Work out the finished part from the listing and answer in its coordinate system (mm). Face numbers are marked on the shaded views. Coordinates: 2 decimals unless noted, no trailing zeros. Loops run counter-clockwise (first coordinate to the right, second up) from the corner with the lowest first, then second, coordinate; pieces in that order, holes last.
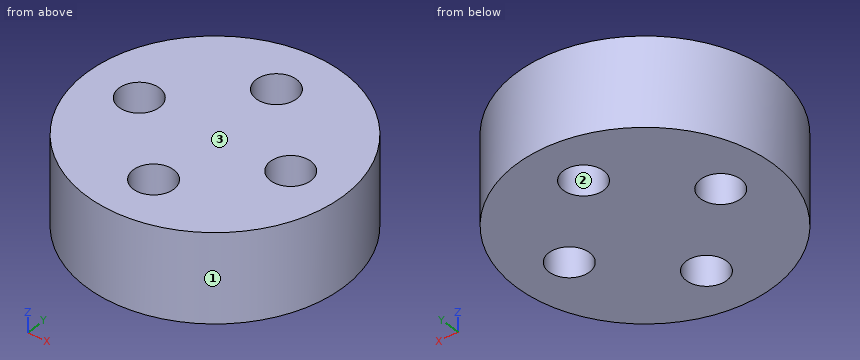
Autodesk Inventor part; units mm, degrees
ref_plane "YZ Plane" through (0, 0, 0) normal (1, 0, 0) x (0, 1, 0)
ref_plane "XZ Plane" through (0, 0, 0) normal (0, 1, 0) x (-1, 0, 0)
ref_plane "XY Plane" through (0, 0, 0) normal (0, 0, 1) x (1, 0, 0)
sketch "스케치1" plane through (0, 0, 0) normal (0, 0, 1) x (1, 0, 0)
  circle A0 centre (0, 0) radius 10.15
  line L0 (0, 0) -> (-6, 0)
  circle A1 centre (-6, 0) radius 1.6
  line L1 (0, 0) -> (0, 6)
  circle A2 centre (0, 6) radius 1.6
  line L2 (0, 0) -> (0, -6)
  circle A3 centre (0, -6) radius 1.6
  line L3 (0, 0) -> (6, 0)
  circle A4 centre (6, 0) radius 1.6
  dimension "d2" = 6
  dimension "d3" = 3.2
  dimension "d7" = 6
  dimension "d8" = 3.2
  dimension "d9" = 6
  dimension "d10" = 3.2
  dimension "d11" = 6
  dimension "d12" = 3.2
  dimension "d13" = 20.3
extrude "돌출1" add sketch "스케치1" along normal blind 6
thicken "두껍게 하기1" operation add thickness 1 both sides no extend neighbours no toward (0, 0, 1) faces at (-0.0643, -1.4706, 6)
equation "\"d5\" = d7"
properties part number "Test_ShaftB"
1. Determine the mould class of the marked faces 1, 2 and 3 for opening direction Y: released by +Y, released by -Y, zero draft, split by the parting line, or undercut.
2. A cutting plane is placed at D-D, the plane x = 6. Give the vertices of the cut face in (y, z), then the cut area to 3 significant figures.
3. A cutting plane is placed at C-C, the plane z = 6.25. Give the vertices of the cut face in (x, y), then the cut area to 3 significant figures.
4. Straight lines are drawn through the part: probe 1 along Y at (x, z) = (0, 1.75); probe 2 along Y at (x, z) = (1.25, 6.25); probe 3 along Y at (x, z) = (6, 5.25). For each, find the intervals that lie inside material, in ascending order.
5. Each of these flat-tipped pins is pushed along its axis until it touches: P1, Ø3, axis at x = 6, y = 6.5, coming from the -Z side; P2, Ø2.5, axis at x = 0, y = 6, coming from the -Z side; P3, Ø2, axis at x = 5.5, z = 4.5, coming from the -Y side. Where does it stop, or does it pass through?
6. A cutting plane is placed at A-A, the plane y = 0. Give the vertices of the cut face in (x, z), then the cut area to 3 significant figures.
Answers below:
1. face 1: split by the parting line
1. face 2: undercut
1. face 3: zero draft
2. outline: (-8.19, 0) - (-1.6, 0) - (-1.6, 7) - (-8.19, 7) - close; (1.6, 0) - (8.19, 0) - (8.19, 7) - (1.6, 7) - close
2. area: 92.2 mm2
3. outline: circle Ø20.3 at (0, 0); hole circle Ø3.2 at (-6, 0); hole circle Ø3.2 at (0, -6); hole circle Ø3.2 at (0, 6); hole circle Ø3.2 at (6, 0)
3. area: 291 mm2
4. probe 1: y = -10.15 to -7.6, -4.4 to 4.4, 7.6 to 10.15
4. probe 2: y = -10.07 to -7, -5 to 5, 7 to 10.07
4. probe 3: y = -8.19 to -1.6, 1.6 to 8.19
5. P1: stops at z = 0
5. P2: passes through
5. P3: stops at y = -9.1
6. outline: (-10.15, 0) - (-7.6, 0) - (-7.6, 7) - (-10.15, 7) - close; (-4.4, 0) - (4.4, 0) - (4.4, 7) - (-4.4, 7) - close; (7.6, 0) - (10.15, 0) - (10.15, 7) - (7.6, 7) - close
6. area: 97.3 mm2
